from build123d import *

# Parameters (mm, degrees)
PAD_DEPTH    = 90
SKETCH001_R  = 3
POCKET_DEPTH = 5
FILLET_R     = 15
FILLET001_R  = 1
FILLET002_R  = 1


with BuildPart() as part:
    # Sketch (on XY_Plane of Origin) → Pad (new body)
    with BuildSketch(Plane.XY):
        with BuildLine():
            Line((-49.441831, 0), (-5, 0))
            Line((-5, 0), (0, 5))
            Line((0, 5), (0, 8.139563))
            Line((0, 8.139563), (0, 34.804017))
            Line((0, 34.804017), (-5, 39.804017))
            Line((-5, 39.804017), (-25.687218, 39.804017))
            Line((-25.687218, 39.804017), (-25.687218, 34.804017))
            Line((-10, 34.804017), (-25.687218, 34.804017))
            ThreePointArc((-5, 29.804017), (-6.464466, 33.339551), (-10, 34.804017))
            Line((-5, 10), (-5, 29.804017))
            ThreePointArc((-10, 5), (-6.464466, 6.464466), (-5, 10))
            Line((-20, 5), (-10, 5))
            Line((-20, 5), (-49.441831, 5))
            Line((-49.441831, 5), (-49.441831, 0))
        make_face()
    extrude(amount=PAD_DEPTH)

    # Sketch001 → Pocket (cut)
    with BuildSketch(Plane(origin=(0, 5, 0), x_dir=(-1, 0, 0), z_dir=(0, 1, 0))):
        with Locations((38.441831, 80.5)):
            Circle(SKETCH001_R)
        with Locations((38.441831, 9.5)):
            Circle(SKETCH001_R)
    extrude(amount=-POCKET_DEPTH, mode=Mode.SUBTRACT)

    # Fillet
    fillet_edges = [part.edges().sort_by_distance(p)[0] for p in [
        (-25.687218, 37.304017, 90),
        (-25.687218, 37.304017, 0),
        (-49.441831, 2.5, 0),
        (-49.441831, 2.5, 90),
    ]]
    fillet(fillet_edges, radius=FILLET_R)

    # Fillet001
    fillet001_edges = [part.edges().sort_by_distance(p)[0] for p in [
        (-49.441831, 5, 45),
        (-45.048433, 5, 85.606602),
        (-22.220916, 5, 90),
        (-45.048433, 5, 4.393398),
        (-22.220916, 5, 0),
    ]]
    fillet(fillet001_edges, radius=FILLET001_R)

    # Fillet002
    fillet002_edges = [part.edges().sort_by_distance(p)[0] for p in [
        (-21.29382, 39.804017, 85.606602),
        (-25.687218, 39.804017, 45),
        (-21.29382, 39.804017, 4.393398),
    ]]
    fillet(fillet002_edges, radius=FILLET002_R)


solid = part.part
Model file for the job. Use its own axes, mm. A direction names the side the tool comes from. Give positions to 0.01 mm unless a question says otherwise; leave off trailing zeros. Write each loop counter-clockwise with the first axis right and the second up, starting at its lowest first coordinate (ties: lowest second). Pieces come first, ordered by that corner, then holes. Notation, with made-up numbers: M -0.75,-19.5 L 32.25,-19.5 A29 cw 32.25,13.5 Z; hole C 21,79 d7. An arc over 180 degrees is marked long. One line per item, written item: value. Start each with the question number.
Q1. Saw through at B-B, the plane x = -28. Write the cut outline in (y, z).
Q2. Saw through at D-D, the plane x = -40. State how many separate pieces and enclosed holes the cut face has, plus the area to 3 significant figures.
Q3. Saw through at A-A, the plane z = 51. Write the cut outline in (x, y), plus the area to 3 significant figures.
Q4. 3-axis set-ups, long thin cutter, end or side, ignore diameter. For faces 4 (the flat face through (-25.687, 37, 45)), 5 (the cylindrical face through (-21.2, 37.3, 85.7)), 6 (the cylindrical face through (-21.2, 37.3, 4.3)), 7 (the cylindrical face through (-6.426, 33.3, 44.384)): which of +Z, -Z, +X, -X, +Y, -Y reach the whole face in a straight line?
Q5. Saw through at C-C, the plane y = 25.5. Write the cut outline in (x, z), plus the area to 3 significant figures.
Q6. Two-plate mould, pull along Y, no slides. Class faces 1 (the flat face through (-28, 0, 44)), 2 (the flat face through (0, 20, 44)), 3 (the flat face through (-29, 5, 44)): +Y half, -Y half, draft (parallel to the pull), parting line (faces both ways), or undercut.
Q7. Probe probe 1 along Y at (x, z) = (-11.5, 57); probe 2 along Y at (x, z) = (-25.5, 34.5); probe 3 along Y at (x, z) = (-42.5, 17). List the from-to ranges inside material, lowest first. Write a range as [from, to].
Q8. Drop flat-ended pins along their axis: pin 1 Ø5.5 at (x, z) = (-38.44, 80.5) entering from -Y; pin 2 Ø22 at (y, z) = (15.5, 39) entering from -X; pin 3 Ø3.5 at (y, z) = (37, 45) entering from -X; pin 4 Ø1.5 at (x, y) = (-5, 29.5) entering from +Z. Give the stop position or say it passes through.
Output values:
1. outline: M 0,0 L 4,0 A1 ccw 5,1 L 5,89 A1 ccw 4,90 L 0,90 Z
2. separate pieces: 3
2. enclosed holes: 0
2. area: 388 mm²
3. outline: M -49.44,0 L -5,0 L 0,5 L 0,34.8 L -5,39.8 L -24.69,39.8 A1 ccw -25.69,38.8 L -25.69,35.8 A1 ccw -24.69,34.8 L -10,34.8 A5 cw -5,29.8 L -5,10 A5 cw -10,5 L -48.44,5 A1 ccw -49.44,4 Z
3. area: 510 mm²
4. face 4: +Z, -Z, -X, +Y
4. face 5: +Z, -X, +Y
4. face 6: -Z, -X, +Y
4. face 7: +Z, -Z, -X
5. outline: M -5,1 A1 ccw -4,0 L 0,0 L 0,90 L -4,90 A1 ccw -5,89 Z
5. area: 450 mm²
6. face 1: -Y half
6. face 2: draft
6. face 3: undercut
7. probe 1: y = [0, 5], [34.8, 39.8]
7. probe 2: y = [0, 5], [35.22, 39.39]
7. probe 3: y = [0, 5]
8. pin 1: passes through
8. pin 2: stops at x = -49.31
8. pin 3: stops at x = -25.69
8. pin 4: stops at z = 89.97
